Design review of the part built by this model. Coordinates are the model's own, in mm. A direction names the side the tool comes from. Round coordinates to 2 decimals unless told otherwise and drop trailing zeros. Order: outer loops, then holes, each group sorted by start corner. A loop starts at its lowest first (then second) coordinate and runs counter-clockwise, first axis right, second up. Notation, with made-up numbers: (-23, 30) - (-6, 30) arc R21 cw to (-6, 65) - close; hole circle Ø7 at (-30, -15.5). An arc over 180 degrees is marked (long way). Use CSV: the item, a comma, the result in double quotes.
from build123d import *

# Parameters (mm, degrees)
SKETCH_1_R      = 1.75
EXTRUDE_1_DEPTH = 1.5
SKETCH_2_W      = 13.622112507
SKETCH_2_H      = 2.131934571
EXTRUDE_2_DEPTH = 2


with BuildPart() as part:
    # 草图1 → 凸台-拉伸1 (new body)
    with BuildSketch(Plane(origin=(0, 0, 0), x_dir=(1, 0, 0), z_dir=(0, 1, 0))):
        with BuildLine():
            Line((-7.23910046, -7.314129875), (-7.23910046, -17.924733935))
            Line((-7.23910046, -17.924733935), (18.76089954, -17.924733935))
            Line((18.76089954, -17.924733935), (18.76089954, -15.792799364))
            Line((18.76089954, -15.792799364), (5.138787033, -15.792799364))
            Line((5.138787033, -15.792799364), (5.138787033, -8.792799364))
            ThreePointArc((5.138787033, -8.792799364), (9.069997492, -5.118417293), (10.730510575, 0))
            ThreePointArc((10.730510575, 0), (7.980510575, 2.75), (5.230510575, 0))
            ThreePointArc((5.230510575, 0), (-0.009744712, -5.827408606), (-5.25, 0))
            ThreePointArc((-5.25, 0), (-8, 2.75), (-10.75, 0))
            ThreePointArc((-10.75, 0), (-9.710304188, -4.000638307), (-7.23910046, -7.314129875))
        make_face()
        with Locations(Location((-8, 0, 0), (0, 0, 270))):
            Circle(SKETCH_1_R, mode=Mode.SUBTRACT)
        with Locations(Location((8, 0, 0), (0, 0, 270))):
            Circle(SKETCH_1_R, mode=Mode.SUBTRACT)
    extrude(amount=EXTRUDE_1_DEPTH)

    # 草图2 → 凸台-拉伸2 (add)
    with BuildSketch(Plane(origin=(0, 1.5, 0), x_dir=(1, 0, 0), z_dir=(0, 1, 0))):
        with Locations((11.949843287, -16.85876665)):
            Rectangle(SKETCH_2_W, SKETCH_2_H)
    extrude(amount=EXTRUDE_2_DEPTH)


solid = part.part
1) We need section D-D (x = 12.5). Give the boundary of the cut face in (y, z), then the cut area to 3 significant figures.
Data:
outline,"(0, 15.79) - (3.5, 15.79) - (3.5, 17.92) - (0, 17.92) - close"
area,"7.46 mm2"
2) Insertion check: pin 1 Ø1.2 at (y, z) = (0.5, 13) entering from +X; pin 2 Ø4.5 at (x, z) = (8, 0) entering from +Y; pin 3 Ø8.5 at (x, z) = (-0.01, 0.56) entering from -Y; pin 4 Ø0.6 at (y, z) = (3, 17) entering from -X. Each pin has a flat end and moves straight along its axis. Give the tip position at first contact, or say it passes through.
Data:
pin 1,"stops at x = 5.14"
pin 2,"stops at y = 1.5"
pin 3,"passes through"
pin 4,"stops at x = 5.14"
3) We need section B-B (z = 1). Give the boundary of the cut face in (x, y), then the cut area to 3 significant figures.
Data:
outline,"(-10.64, 0) - (-9.44, 0) - (-9.44, 1.5) - (-10.64, 1.5) - close; (-6.56, 0) - (-5.26, 0) - (-5.26, 1.5) - (-6.56, 1.5) - close; (5.24, 0) - (6.56, 0) - (6.56, 1.5) - (5.24, 1.5) - close; (9.44, 0) - (10.62, 0) - (10.62, 1.5) - (9.44, 1.5) - close"
area,"7.53 mm2"
4) The part is to be moulded in two halves that separate along X. For faces 5 (the face through (5.139, 1, 12)), 6 (the face through (-9.735, 0.74, 3.948)), 7 (the face through (-9.55, 0.74, 0.81)), 8 (the face through (-7.94, 0.74, -2.75)), say which applies: +X half, -X half, draft (parallel to the pull), parting line (faces both ways), or undercut.
Data:
face 5,"+X half"
face 6,"-X half"
face 7,"undercut"
face 8,"undercut"
5) We need section A-A (x = 7.5). Give the boundary of the cut face in (y, z).
Data:
outline,"(0, -2.71) - (1.5, -2.71) - (1.5, -1.68) - (0, -1.68) - close; (0, 1.68) - (1.5, 1.68) - (1.5, 7.05) - (0, 7.05) - close; (0, 15.79) - (3.5, 15.79) - (3.5, 17.92) - (0, 17.92) - close"
6) For faces 1 (the face through (9.03, 0.74, 5.18)), 2 (the face through (5.139, 2, 17)), 3 (the face through (-7.239, 1, 13)), 4 (the face through (0, 1.5, 7)), list the 3-axis set-ups (+Z, -Z, +X, -X, +Y, -Y) from which the entire face can be reached by the end or side of a thin tool; tool diameter is ignored.
Data:
face 1,"+X, +Y, -Y"
face 2,"+Z, -Z, -X, +Y"
face 3,"+Z, -X, +Y, -Y"
face 4,"-Z, -X, +Y"
7) To check wall thickness, follow L1, parallel to X at y = 0.7, z = 0.5; L2, parallel to X at y = 1, z = 14; L3, parallel to Y at x = 4, z = 6.75. State the ranges of each line that lie inside material, in increasing order. Write a range as from..to.
Data:
L1,"x = -10.71..-9.68, -6.32..-5.28, 5.26..6.32, 9.68..10.69"
L2,"x = -7.24..5.14"
L3,"y = 0..1.5"
8) We need section C-C (x = -8). Give the boundary of the cut face in (y, z).
Data:
outline,"(0, -2.75) - (1.5, -2.75) - (1.5, -1.75) - (0, -1.75) - close; (0, 1.75) - (1.5, 1.75) - (1.5, 6.55) - (0, 6.55) - close"
